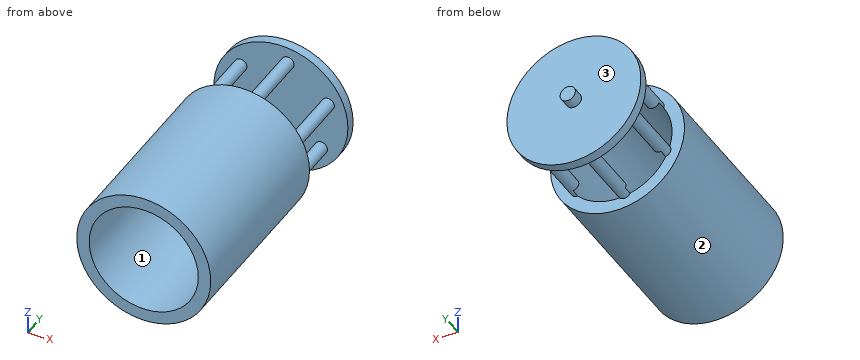
```python
from build123d import *

# Parameters (mm, degrees)
SKETCH1_R           = 27.955
BOSS_EXTRUDE1_DEPTH = 4
SKETCH2_R           = 3.175
BOSS_EXTRUDE2_DEPTH = 4.76
SKETCH3_R           = 2.615316251
BOSS_EXTRUDE3_DEPTH = 29.718
SKETCH4_R           = 27.955
BOSS_EXTRUDE4_DEPTH = 76.35
SKETCH5_R           = 22.758745994
CUT_EXTRUDE1_DEPTH  = 80


with BuildPart() as part:
    # Sketch1 → Boss-Extrude1 (new body)
    with BuildSketch(Plane(origin=(0, 0, 0), x_dir=(1, 0, 0), z_dir=(0, 1, 0))):
        Circle(SKETCH1_R)
    extrude(amount=BOSS_EXTRUDE1_DEPTH)

    # Sketch2 → Boss-Extrude2 (add)
    with BuildSketch(Plane(origin=(0, 4, 0), x_dir=(1, 0, 0), z_dir=(0, 1, 0))):
        Circle(SKETCH2_R)
    extrude(amount=BOSS_EXTRUDE2_DEPTH)

    # Sketch3 → Boss-Extrude3 (add)
    with BuildSketch(Plane.XZ):
        with Locations((2.874048201, 21.060648295)):
            Circle(SKETCH3_R)
        with Locations((19.676080545, 8.041325394)):
            Circle(SKETCH3_R)
        with Locations((16.802032343, -13.019322902)):
            Circle(SKETCH3_R)
        with Locations((-2.874048201, -21.060648295)):
            Circle(SKETCH3_R)
        with Locations((-19.676080545, -8.041325394)):
            Circle(SKETCH3_R)
        with Locations((-16.802032343, 13.019322902)):
            Circle(SKETCH3_R)
    extrude(amount=BOSS_EXTRUDE3_DEPTH)

    # Sketch4 → Boss-Extrude4 (add)
    with BuildSketch(Plane.XZ.offset(29.718)):
        Circle(SKETCH4_R)
    extrude(amount=BOSS_EXTRUDE4_DEPTH)

    # Sketch5 → Cut-Extrude1 (cut)
    with BuildSketch(Plane.XZ.offset(106.068)):
        Circle(SKETCH5_R)
    extrude(amount=-CUT_EXTRUDE1_DEPTH, mode=Mode.SUBTRACT)


solid = part.part
```
The model under review builds one solid part; all positions refer to its coordinate system, in mm. Face numbers are marked on the shaded views. Round coordinates to 2 decimals unless told otherwise and drop trailing zeros. Order: outer loops, then holes, each group sorted by start corner. A loop starts at its lowest first (then second) coordinate and runs counter-clockwise, first axis right, second up. Notation, with made-up numbers: (52.5, 57) - (66.5, 57) arc R23 cw to (66.5, 73) - close; hole circle Ø1 at (67.25, 63.5). An arc over 180 degrees is marked (long way). Answer in a Markdown table with one row per item.
(1) For line 1 (Y direction, x = -2.5, z = -24); line 2 (Z direction, x = 0, y = -74) (3 decimals); line 3 (Z direction, x = -1, y = -77.5), list the stretches that pass through material, from the lowest coordinate up. Write a range as from..to.
Result set:
| item | result |
|---|---|
| line 1 | y = -106.07..-29.72, 0..4 |
| line 2 | z = -27.955..-22.759, 22.759..27.955 |
| line 3 | z = -27.94..-22.74, 22.74..27.94 |
(2) Take a section at C-C on y = -81.5. Write out the cut boundary in (x, z) (1 decimal), plus the area to 3 significant figures.
Result set:
| item | result |
|---|---|
| outline | circle Ø55.9 at (0, 0); hole circle Ø45.5 at (0, 0) |
| area | 828 mm2 |
(3) Mouldability with a two-part tool opening along Z and no side actions: class the marked faces 1, 2 and 3 as released by +Z, released by -Z, zero draft, split by the parting line, or undercut.
Result set:
| item | result |
|---|---|
| face 1 | undercut |
| face 2 | split by the parting line |
| face 3 | zero draft |
(4) Clearance check with flat-ended pins moving along their axes: P1, Ø8, axis at x = 9.5, z = 6, coming from the +Y side; P2, Ø1.5, axis at y = -81.5, z = 8.5, coming from the -X side; P3, Ø5, axis at x = -4, z = 5, coming from the -Y side. State where each tip first meets the part, or that it passes through.
Result set:
| item | result |
|---|---|
| P1 | stops at y = 4 |
| P2 | stops at x = -26.86 |
| P3 | stops at y = 0 |
(5) Take a section at B-B on x = -9.5. Write out the cut boundary in (y, z), plus the area to 3 significant figures.
Result set:
| item | result |
|---|---|
| outline | (-106.07, -26.29) - (-29.72, -26.29) - (-29.72, -20.68) - (-106.07, -20.68) - close; (-106.07, 20.68) - (-29.72, 20.68) - (-29.72, 26.29) - (-106.07, 26.29) - close; (0, -26.29) - (4, -26.29) - (4, 26.29) - (0, 26.29) - close |
| area | 1,070 mm2 |
(6) Take a section at A-A on z = 0. Write out the cut boundary in (x, y) (3 decimals).
Result set:
| item | result |
|---|---|
| outline | (-27.955, -106.068) - (-22.759, -106.068) - (-22.759, -29.718) - (-27.955, -29.718) - close; (-27.955, 0) - (27.955, 0) - (27.955, 4) - (3.175, 4) - (3.175, 8.76) - (-3.175, 8.76) - (-3.175, 4) - (-27.955, 4) - close; (22.759, -106.068) - (27.955, -106.068) - (27.955, -29.718) - (22.759, -29.718) - close |
